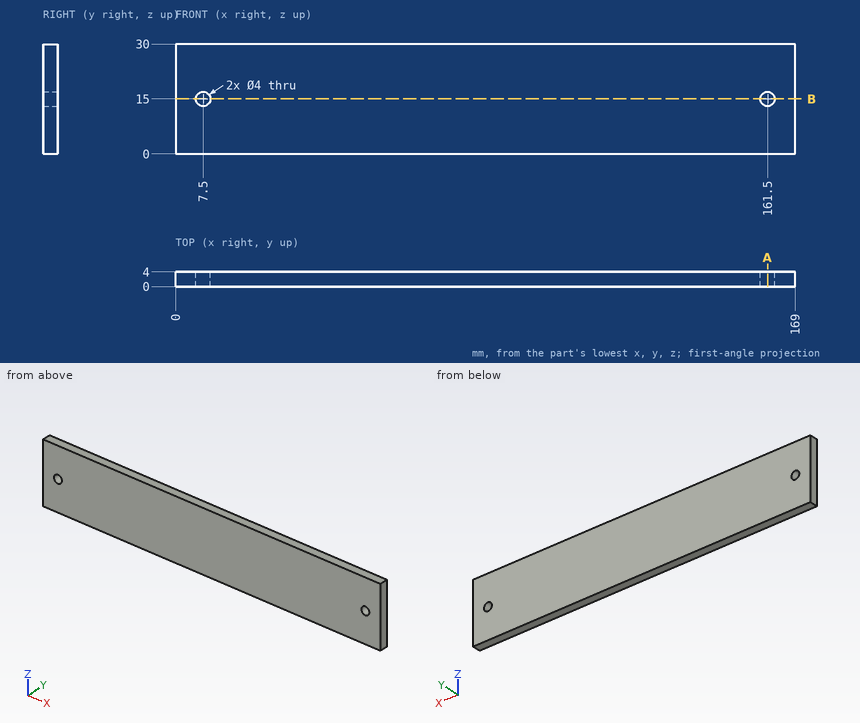
Verification items for this drawing (mm, ordinates from the low corner). Coordinates: 2 decimals unless noted, no trailing zeros. Loops run counter-clockwise (first coordinate to the right, second up) from the corner with the lowest first, then second, coordinate; pieces in that order, holes last. Notation, with made-up numbers: (-2, 24.25) -> (31, 24.25) arc R12 ccw to (31, 33.25) -> close; hole circle Ø8 at (-34, 40.25). An arc over 180 degrees is marked (long way). Answer in a Markdown table with one row per item. Add a question column.
1. Section check A-A, the plane x = 161.5. Enter the section's corners in (y, z), then the cut area to 3 significant figures.
2. Depth check by flat-ended pin: P1, Ø6.5, axis at x = 161.5, z = 15, coming from the -Y side. Enter the tip coordinate at first touch or a pass-through.
3. Section check B-B, the plane z = 15. Enter the section's corners in (x, y), then the cut area to 3 significant figures.
4. Material ranges on probe 1 along X at (y, z) = (2.7, 15); probe 2 along Z at (x, y) = (161.5, 2.8), recorded low to high. Write a range as [from, to].
Derived:
| question | item | result |
|---|---|---|
| 1 | outline | (0, 0) -> (4, 0) -> (4, 13) -> (0, 13) -> close; (0, 17) -> (4, 17) -> (4, 30) -> (0, 30) -> close |
| 1 | area | 104 mm² |
| 2 | P1 | stops at y = 0 |
| 3 | outline | (0, 0) -> (5.5, 0) -> (5.5, 4) -> (0, 4) -> close; (9.5, 0) -> (159.5, 0) -> (159.5, 4) -> (9.5, 4) -> close; (163.5, 0) -> (169, 0) -> (169, 4) -> (163.5, 4) -> close |
| 3 | area | 644 mm² |
| 4 | probe 1 | x = [0, 5.5], [9.5, 159.5], [163.5, 169] |
| 4 | probe 2 | z = [0, 13], [17, 30] |
